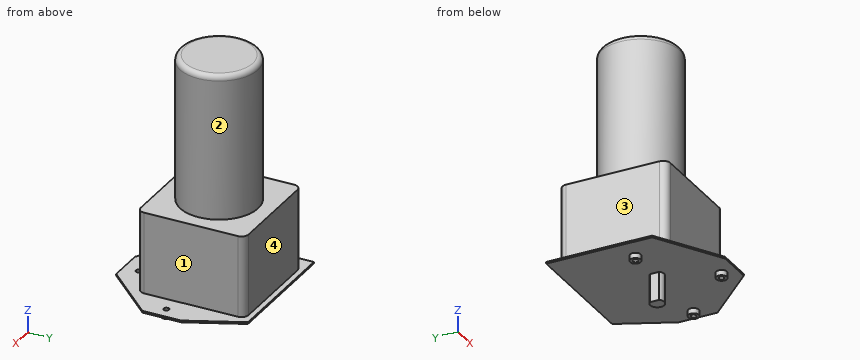
Autodesk Fusion 360 part; units mm, degrees
sketch "Esboço1" plane through (0, 0, 0) normal (0, 0, 1) x (1, 0, 0)
  line L0 (30.5, -30.5) -> (-30.5, -30.5)
  line L1 (-30.5, -30.5) -> (-30.5, 30.5)
  line L2 (-30.5, 30.5) -> (30.5, 30.5)
  line L3 (30.5, 30.5) -> (30.5, -30.5)
  line L4 (30.5, -30.5) -> (-30.5, 30.5) construction
  line L5 (-30.5, -30.5) -> (30.5, 30.5) construction
  circle A0 centre (0, 0) radius 22.075
  dimension "d1" = 61
  dimension "d2" = 44.15
extrude "Extrusão1" add sketch "Esboço1" along normal blind 46.1
extrude "Extrusão2" add sketch "Esboço1" along normal blind 128.3 contours A0
fillet "Arredondamento1" radius 4 4 edges at (30.5, -30.5, 23.05) (30.5, 30.5, 23.05) (-30.5, 30.5, 23.05) (-30.5, -30.5, 23.05)
fillet "Arredondamento2" radius 3 1 edges at (-20.5811, -7.9827, 128.3)
sketch "Esboço3" plane through (0, 0, 0) normal (0, 0, 1) x (1, 0, 0)
sketch "Esboço4" plane through (0, 0, 0) normal (0, 0, 1) x (1, 0, 0)
  line L0 (-38.1983, -26.2505) -> (-1.3738, -48.4531)
  line L1 (-1.3738, -48.4531) -> (18.8762, -48.4531)
  line L2 (18.8762, -48.4531) -> (47.1993, -18.8085)
  line L3 (47.1993, -18.8085) -> (47.1993, 3.1915)
  line L4 (47.1993, 3.1915) -> (33.3001, 33.6725)
  line L5 (33.3001, 33.6725) -> (-38.1999, 33.6725)
  line L6 (-38.1999, 33.6725) -> (-38.1983, -26.2505)
  circle A0 centre (-25, -10) radius 1.5
  circle A1 centre (11, -40) radius 1.5
  circle A2 centre (40, -9) radius 1.5
  circle A3 centre (11, -40) radius 3
  circle A4 centre (40, -9) radius 3
  circle A5 centre (-25, -10) radius 3
  dimension "d25" = 3
  dimension "d26" = 3
  dimension "d27" = 3
  dimension "d28" = 20.25
  dimension "d29" = 43
  dimension "d30" = 71.5
  dimension "d31" = 33.5004
  dimension "d32" = 22
  dimension "d33" = 41
  dimension "d38" = 6
  dimension "d39" = 6
  dimension "d40" = 6
extrude "Extrusão5" add sketch "Esboço4" against normal blind 1 contours L0 L1 L2 L3 L4 L5 L6 | A3 | A4 | A5
extrude "Extrusão6" add sketch "Esboço4" against normal blind 4 contours A3 | A4 | A5
sketch "Esboço5" plane through (0, 0, -1) normal (0, 0, -1) x (1, 0, 0)
  circle A0 centre (40, 9) radius 3
  circle A1 centre (-25, 10) radius 3
  circle A2 centre (11, 40) radius 3
  line L0 (-38.1983, 26.2505) -> (-38.1999, -33.6725)
  line L1 (-38.1999, -33.6725) -> (33.3001, -33.6725)
  line L2 (33.3001, -33.6725) -> (47.1993, -3.1915)
  line L3 (47.1993, -3.1915) -> (47.1993, 18.8085)
  line L4 (47.1993, 18.8085) -> (18.8762, 48.4531)
  line L5 (18.8762, 48.4531) -> (-1.3738, 48.4531)
  line L6 (-1.3738, 48.4531) -> (-38.1983, 26.2505)
  line L7 (-1.3738, 48.4531) -> (-1.3738, 10) construction
  line L8 (-1.3738, 10) -> (-25, 10) construction
  line L9 (-5.3738, 10) -> (-4.3738, 10) construction
  line L10 (-4.3738, 10) -> (-4.3738, 7.3542)
  line L11 (-4.3738, 10) -> (-4.3738, 12.6458)
  arc A3 (-4.3738, 7.3542) -> (-4.3738, 12.6458) centre (-1.3738, 10) ccw
  dimension "d47" = 8
  dimension "d48" = 1
extrude "Extrusão8" add sketch "Esboço5" along normal blind 16 contours L10 L11 A3
equation "d5 = 46.1 mm + 82.2 mm"
The model under review builds one solid part; all positions refer to its coordinate system, in mm. Face numbers are marked on the shaded views. A direction names the side the tool comes from. Round coordinates to 2 decimals unless told otherwise and drop trailing zeros. Loops run counter-clockwise (first coordinate to the right, second up) from the corner with the lowest first, then second, coordinate; pieces in that order, holes last. Notation, with made-up numbers: (49.25, 29.25) -> (80.25, 29.25) arc R26 cw to (80.25, 66.25) -> close; hole circle Ø8 at (25.5, 78.5). An arc over 180 degrees is marked (long way). Answer as a JSON object with one key per item and string values. Group by question number.
1) For the marked faces 1, 2, 3 and 4, list the 3-axis set-ups (+Z, -Z, +X, -X, +Y, -Y) from which the entire face can be reached by the end or side of a thin tool; tool diameter is ignored.
2) For line 1 (Y direction, x = 11, z = -2); line 2 (Y direction, x = 40, z = -2); line 3 (Z direction, x = 7.5, y = -17.5), list the stretches that pass through material, from the lowest coordinate up. Write a range as [from, to].
3) We need section B-B on x = 25. Write out the cut boundary in (y, z).
4) We need section C-C on y = 0. Write out the cut boundary in (x, z) (3 decimals).
5) We need section A-A on z = 41.5. Write out the cut boundary in (x, y), then the cut area to 3 significant figures.
6) For pin 1 Ø1.8 at (x, y) = (10, -40.5) entering from -Z; pin 2 Ø2.5 at (x, y) = (11, -40) entering from -Z; pin 3 Ø6 at (x, z) = (-24, 16.5) entering from -Y; pin 4 Ø1 at (x, y) = (4, -33) entering from -Z, all flat-tipped, find the tip position at first contact; note any pin that passes through.
7) We need section D-D on z = 79. Write out the cut boundary in (x, y) (3 decimals), then the cut area to 3 significant figures.
Result set:
{
 "1": {"face 1": "+Z, +X, +Y, -Y", "face 2": "+Z", "face 3": "+Z, -X, +Y, -Y", "face 4": "+Z, +X, -X, +Y"},
 "2": {"line 1": "[-43, -41.5], [-38.5, -37]", "line 2": "[-12, -10.5], [-7.5, -6]", "line 3": "[-1, 128.3]"},
 "3": {"outline": "(-42.04, -1) -> (33.67, -1) -> (33.67, 0) -> (30.5, 0) -> (30.5, 46.1) -> (-30.5, 46.1) -> (-30.5, 0) -> (-42.04, 0) -> close"},
 "4": {"outline": "(-38.199, -1) -> (47.199, -1) -> (47.199, 0) -> (30.5, 0) -> (30.5, 46.1) -> (22.075, 46.1) -> (22.075, 125.3) arc R3 ccw to (19.075, 128.3) -> (-19.075, 128.3) arc R3 ccw to (-22.075, 125.3) -> (-22.075, 46.1) -> (-30.5, 46.1) -> (-30.5, 0) -> (-38.199, 0) -> close"},
 "5": {"outline": "(-30.5, -26.5) arc R4 ccw to (-26.5, -30.5) -> (26.5, -30.5) arc R4 ccw to (30.5, -26.5) -> (30.5, 26.5) arc R4 ccw to (26.5, 30.5) -> (-26.5, 30.5) arc R4 ccw to (-30.5, 26.5) -> close", "area": "3,710 mm²"},
 "6": {"pin 1": "z = -4", "pin 2": "through", "pin 3": "y = -30.5", "pin 4": "z = -1"},
 "7": {"outline": "circle Ø44.15 at (0, 0)", "area": "1,530 mm²"}
}
